Input: part model. Units: mm. Frame: model coordinates. Face numbers are marked on the shaded views. Coordinates: 2 decimals unless noted, no trailing zeros. Write each loop counter-clockwise with the first axis right and the second up, starting at its lowest first coordinate (ties: lowest second). Pieces come first, ordered by that corner, then holes. Notation, with made-up numbers: (14, 40.25) -> (72, 40.25) arc R30 cw to (72, 68.25) -> close; hole circle Ø2 at (-25, 67.5). An arc over 180 degrees is marked (long way). One line per question, with ' | ' between items. Start each with the question number.
```python
from build123d import *

# Parameters (mm, degrees)
SKETCH1_W           = 42
SKETCH1_H           = 62
SKETCH1_R           = 4.15
BOSS_EXTRUDE1_DEPTH = 10
FILLET1_R           = 3
SKETCH2_R           = 2.6
CUT_EXTRUDE1_DEPTH  = 11


with BuildPart() as part:
    # Sketch1 → Boss-Extrude1 (new body)
    with BuildSketch(Plane.XY):
        with Locations((21, 31)):
            Rectangle(SKETCH1_W, SKETCH1_H)
        with Locations((21, 42)):
            Circle(SKETCH1_R, mode=Mode.SUBTRACT)
    extrude(amount=BOSS_EXTRUDE1_DEPTH)

    # Fillet1
    fillet1_edges = [part.edges().sort_by_distance(p)[0] for p in [
        (0, 62, 5),
        (42, 62, 5),
    ]]
    fillet(fillet1_edges, radius=FILLET1_R)

    # Sketch2 → Cut-Extrude1 (cut, through all)
    with BuildSketch(Plane.XY.offset(10)):
        with Locations((5, 7.5)):
            Circle(SKETCH2_R)
        with Locations((21, 7.5)):
            Circle(SKETCH2_R)
        with Locations((37, 7.5)):
            Circle(SKETCH2_R)
    extrude(amount=-CUT_EXTRUDE1_DEPTH, mode=Mode.SUBTRACT)


solid = part.part
```
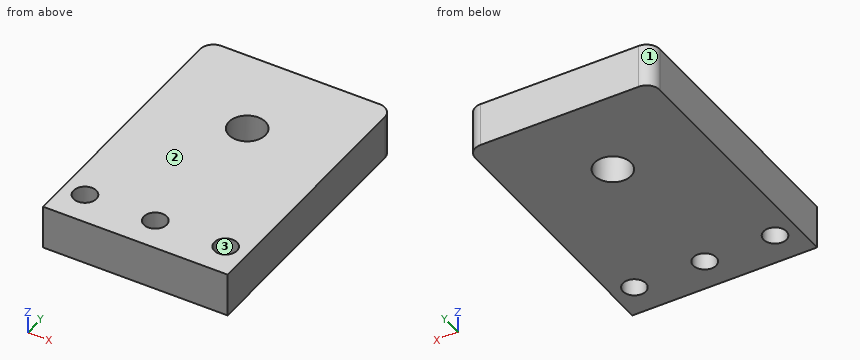
1) Section C-C, the plane z = 3.75. Return loops of the section in (x, y), then the cut area to 3 significant figures.
2) Pull-direction query (Y, two-part tool) for the marked faces 1, 2 and 3; classes: released by +Y, released by -Y, zero draft, split by the parting line, or undercut.
3) Section D-D, the plane x = 21. Return loops of the section in (y, z).
4) Section A-A, the plane y = 7.5. Return loops of the section in (x, z), then the cut area to 3 significant figures.
5) Ray query, line 1 (Y direction, x = 21, z = 5.25); line 2 (Y direction, x = 5, z = 8.5); line 3 (Y direction, x = 23, z = 3.5). Return the intervals inside material, ascending.
6) Section B-B, the plane x = 5. Return loops of the section in (y, z), then the cut area to 3 significant figures.
7) First-contact query: P1, Ø4.5, axis at x = 21, y = 7.5, coming from the -Z side. Flat tip, straight axial feed; report the tip coordinate or a pass-through.
Answer block:
1) outline: (0, 0) -> (42, 0) -> (42, 59) arc R3 ccw to (39, 62) -> (3, 62) arc R3 ccw to (0, 59) -> close; hole circle Ø5.2 at (5, 7.5); hole circle Ø8.3 at (21, 42); hole circle Ø5.2 at (21, 7.5); hole circle Ø5.2 at (37, 7.5) | area: 2,480 mm2
2) face 1: released by +Y | face 2: zero draft | face 3: undercut
3) outline: (0, 0) -> (4.9, 0) -> (4.9, 10) -> (0, 10) -> close; (10.1, 0) -> (37.85, 0) -> (37.85, 10) -> (10.1, 10) -> close; (46.15, 0) -> (62, 0) -> (62, 10) -> (46.15, 10) -> close
4) outline: (0, 0) -> (2.4, 0) -> (2.4, 10) -> (0, 10) -> close; (7.6, 0) -> (18.4, 0) -> (18.4, 10) -> (7.6, 10) -> close; (23.6, 0) -> (34.4, 0) -> (34.4, 10) -> (23.6, 10) -> close; (39.6, 0) -> (42, 0) -> (42, 10) -> (39.6, 10) -> close | area: 264 mm2
5) line 1: y = 0 to 4.9, 10.1 to 37.85, 46.15 to 62 | line 2: y = 0 to 4.9, 10.1 to 62 | line 3: y = 0 to 5.84, 9.16 to 38.36, 45.64 to 62
6) outline: (0, 0) -> (4.9, 0) -> (4.9, 10) -> (0, 10) -> close; (10.1, 0) -> (62, 0) -> (62, 10) -> (10.1, 10) -> close | area: 568 mm2
7) P1: passes through
